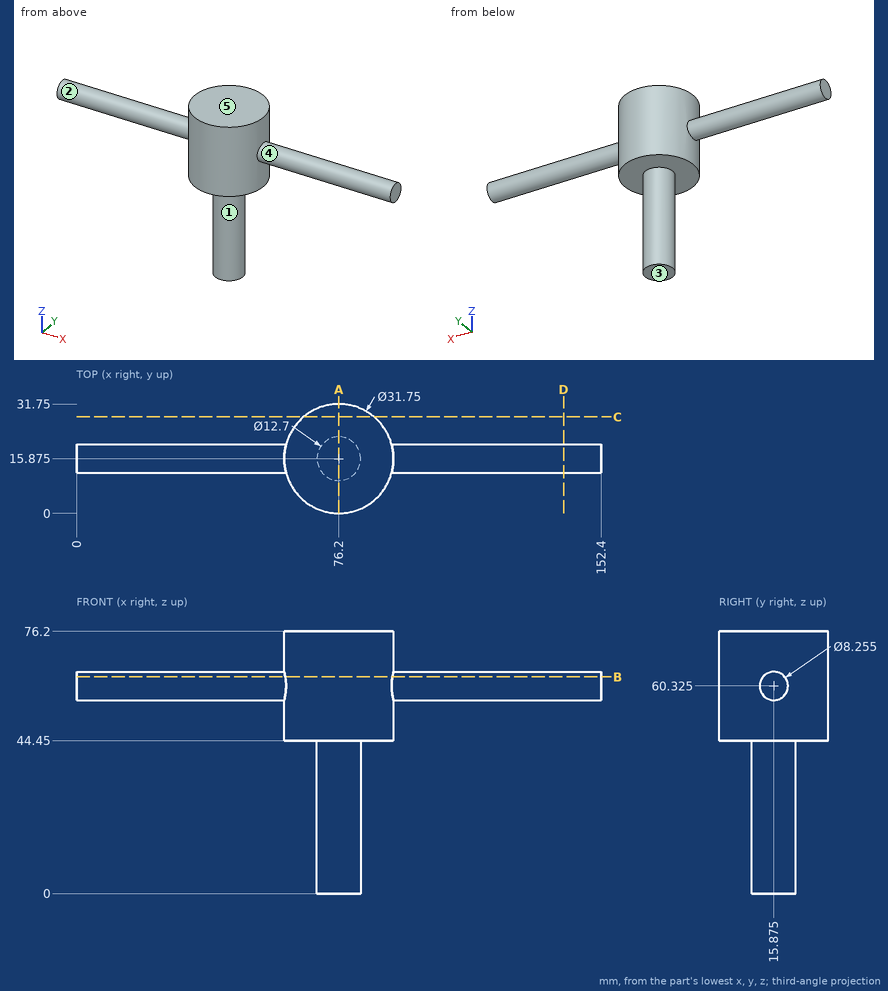
Study the drawing (mm; zero at the part's minimum x, y, z) and answer. A direction names the side the tool comes from. Coordinates: 2 decimals unless noted, no trailing zeros. Write each loop counter-clockwise with the first axis right and the second up, starting at its lowest first coordinate (ties: lowest second). Pieces come first, ordered by that corner, then holes. Notation, with made-up numbers: (-33.5, -16.5) - (-0.5, -16.5) arc R10 cw to (-0.5, -0.5) - close; hole circle Ø11 at (41.25, -38.75). An arc over 180 degrees is marked (long way). Put each result on its own line as item: value.
1. The part is cut by section B-B on z = 63. Give the vertices of the cut face in (x, y) (3 decimals).
Answer sheet:
outline: (0, 12.732) - (60.639, 12.732) arc R15.875 ccw to (91.761, 12.732) - (152.4, 12.732) - (152.4, 19.018) - (91.761, 19.018) arc R15.875 ccw to (60.639, 19.018) - (0, 19.018) - close
2. Flat-ended cylindrical pins translate along their axes: pin 1 Ø1.5 at (y, z) = (9.5, 65.5) entering from +X; pin 2 Ø4 at (x, z) = (81.5, 37) entering from -Y; pin 3 Ø9.5 at (x, y) = (82, 18.5) entering from -Z; pin 4 Ø3 at (x, y) = (83.5, 5) entering from -Z. Find the tip coordinate at first contact, or state that the pin passes through.
Answer sheet:
pin 1: stops at x = 91.05
pin 2: stops at y = 10.45
pin 3: stops at z = 0
pin 4: stops at z = 44.45
3. A tool of negligible diameter and unlimited length cuts with its end or side. For the marked faces 1, 2, 3, 4 and 5, from which of +Z, -Z, +X, -X, +Y, -Y can it reach the whole face along a straight path? Write none if from no direction.
Answer sheet:
face 1: -Z
face 2: -X
face 3: -Z, +X, -X, +Y, -Y
face 4: +X
face 5: +Z, +X, -X, +Y, -Y
4. The part is cut by section D-D on x = 141.5. Give the vertices of the cut face in (y, z) (1 decimal), plus the area to 3 significant figures.
Answer sheet:
outline: circle Ø8.3 at (15.9, 60.3)
area: 53.5 mm^2
5. Find the intervals of material crossed by line 1 along Z through (x, y) = (82.5, 7); line 2 along X through (y, z) = (16.5, 43); line 3 along X through (y, z) = (21, 27), in increasing order. Write a range as from..to.
Answer sheet:
line 1: z = 44.45..76.2
line 2: x = 69.88..82.52
line 3: x = 72.45..79.95
6. The part is cut by section A-A on x = 76.2. Give the vertices of the cut face in (y, z) (3 decimals), plus the area to 3 significant figures.
Answer sheet:
outline: (0, 44.45) - (9.525, 44.45) - (9.525, 0) - (22.225, 0) - (22.225, 44.45) - (31.75, 44.45) - (31.75, 76.2) - (0, 76.2) - close
area: 1,570 mm^2
7. The part is cut by section C-C on y = 28. Give the vertices of the cut face in (x, z).
Answer sheet:
outline: (65.95, 44.45) - (86.45, 44.45) - (86.45, 76.2) - (65.95, 76.2) - close
